from build123d import *

# Parameters (mm, degrees)
SKETCH1_R           = 3.75
BOSS_EXTRUDE1_DEPTH = 18
SKETCH2_W           = 3.535533906
SKETCH2_H           = 3.535533906
CUT_EXTRUDE1_DEPTH  = 10
SKETCH3_W           = 2.1
SKETCH3_H           = 1.45
SKETCH3_H_2         = 2.1
SKETCH3_W_2         = 1.45
CUT_EXTRUDE2_DEPTH  = 8


with BuildPart() as part:
    # Sketch1 → Boss-Extrude1 (new body)
    with BuildSketch(Plane.XY):
        Circle(SKETCH1_R)
    extrude(amount=BOSS_EXTRUDE1_DEPTH)

    # Sketch2 → Cut-Extrude1 (cut)
    with BuildSketch(Plane.XY.offset(18)):
        Rectangle(SKETCH2_W, SKETCH2_H)
    extrude(amount=-CUT_EXTRUDE1_DEPTH, mode=Mode.SUBTRACT)

    # Sketch3 → Cut-Extrude2 (cut)
    with BuildSketch(Plane(origin=(0, 0, 0), x_dir=(-1, 0, 0), z_dir=(0, 0, -1))):
        with Locations((0, 1.775)):
            Rectangle(SKETCH3_W, SKETCH3_H)
        Rectangle(SKETCH3_W, SKETCH3_H_2)
        with Locations((1.775, 0)):
            Rectangle(SKETCH3_W_2, SKETCH3_H_2)
        with Locations((0, -1.775)):
            Rectangle(SKETCH3_W, SKETCH3_H)
        with Locations((-1.775, 0)):
            Rectangle(SKETCH3_W_2, SKETCH3_H_2)
    extrude(amount=-CUT_EXTRUDE2_DEPTH, mode=Mode.SUBTRACT)


solid = part.part
Could you check a few things on this model? Use its own coordinates, in mm. A direction names the side the tool comes from. Coordinates: 2 decimals unless noted, no trailing zeros. Order: outer loops, then holes, each group sorted by start corner. A loop starts at its lowest first (then second) coordinate and runs counter-clockwise, first axis right, second up.
Q1. Suppose I cut it at D-D on x = -3. Please give me the cut outline in (y, z), and give its area (3 significant figures).
Q2. Thinking about a two-plate mould opening in Y: for faces 1 (the flat face through (0, -2, 18)), 2 (the flat face through (-1.05, -2, 4)), which applies, released by +Y, released by -Y, zero draft, split by the parting line, or undercut?
Q3. Will these pins go through, and if not, where does the flat tip stop? pin 1 (1.5 mm diameter, centred on y = 3, z = 9.5, fed in from -X); pin 2 (1.2 mm diameter, centred on y = 2, z = 3.5, fed in from +X); pin 3 (0.8 mm diameter, centred on x = -2, y = 0, fed in from -Z).
Q4. Please list where these lines run through material, in increasing order: L1, parallel to Y at x = 0, z = 14.5; L2, parallel to Y at x = 0, z = 6.5; L3, parallel to X at y = -1.25, z = 10.75.
Q5. Suppose I cut it at A-A on y = 0. Please give me the cut outline in (x, z), and give its area (3 significant figures).
Q6. Suppose I cut it at C-C on z = 13.5. Please give me the cut outline in (x, y), and give its area (3 significant figures).
Q7. Which directions (+Z, -Z, +X, -X, +Y, -Y) give clear straight access to the entire face, cutting with the end or side of a thin tool? Please do faces 3 (the flat face through (0, -1.768, 13)), 4 (the flat face through (-2, 2, 0)), 5 (the flat face through (-2.5, 0, 4)).
Answer:
1. outline: (-2.25, 0) - (2.25, 0) - (2.25, 18) - (-2.25, 18) - close
1. area: 81.0 mm2
2. face 1: zero draft
2. face 2: undercut
3. pin 1: stops at x = -3
3. pin 2: stops at x = 3.48
3. pin 3: stops at z = 8
4. L1: y = -3.75 to -1.77, 1.77 to 3.75
4. L2: y = -3.75 to -2.5, 2.5 to 3.75
4. L3: x = -3.54 to -1.77, 1.77 to 3.54
5. outline: (-3.75, 0) - (-2.5, 0) - (-2.5, 8) - (-1.77, 8) - (-1.77, 18) - (-3.75, 18) - close; (1.77, 8) - (2.5, 8) - (2.5, 0) - (3.75, 0) - (3.75, 18) - (1.77, 18) - close
5. area: 59.6 mm2
6. outline: circle Ø7.5 at (0, 0); hole (-1.77, -1.77) - (1.77, -1.77) - (1.77, 1.77) - (-1.77, 1.77) - close
6. area: 31.7 mm2
7. face 3: +Z
7. face 4: -Z, +X, -X, +Y, -Y
7. face 5: -Z
